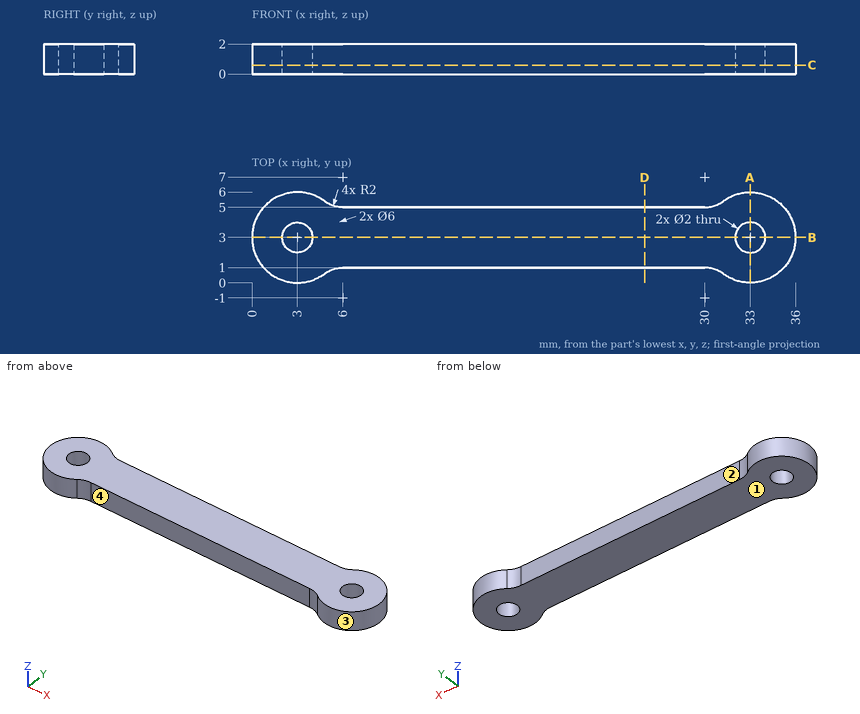
Job drawing, mm, ordinate dimensions from the low corner. One solid piece. A direction names the side the tool comes from. Coordinates: 2 decimals unless noted, no trailing zeros. Write each loop counter-clockwise with the first axis right and the second up, starting at its lowest first coordinate (ties: lowest second). Pieces come first, ordered by that corner, then holes. Notation, with made-up numbers: M -14.5,45 L 24.5,45 A21 cw 24.5,67 Z; hole C 72.25,-23 d9. An arc over 180 degrees is marked long. Answer as a JSON object with one key per item and string values. Group by question number.
1) Pin check, flat tips, straight feed: pin 1 Ø0.6 at (x, z) = (12.5, 1) entering from -Y; pin 2 Ø1 at (y, z) = (1, 0.5) entering from +X; pin 3 Ø1.8 at (x, y) = (33, 3) entering from +Z. Stop position of each tip, or through.
2) Saw through at A-A (x = 33). Write the cut outline in (y, z).
3) Mould opens along X. For the marked faces 1 and 2 say: +X half, -X half, draft (parallel to the pull), parting line (faces both ways), or undercut.
4) Wall check: line 1 (Y direction, x = 3, z = 1.3); line 2 (X direction, y = 3.5, z = 1.65); line 3 (X direction, y = 2.1, z = 1.3). Give the ranges that are in metal, low to high. Write a range as from..to.
5) Saw through at D-D (x = 26). Write the cut outline in (y, z).
6) Tool access for the marked faces 3 and 4: list every direction of +Z, -Z, +X, -X, +Y, -Y with a clear straight run to the whole face (end or side of a thin tool).
7) Saw through at B-B (y = 3). Write the cut outline in (x, z).
8) Saw through at C-C (z = 0.6). Write the cut outline in (x, y), plus the area to 3 significant figures.
Values follow:
{
 "1": {"pin 1": "stops at y = 1", "pin 2": "stops at x = 35.6", "pin 3": "passes through"},
 "2": {"outline": "M 0,0 L 2,0 L 2,2 L 0,2 Z; M 4,0 L 6,0 L 6,2 L 4,2 Z"},
 "3": {"face 1": "draft", "face 2": "undercut"},
 "4": {"line 1": "y = 0..2, 4..6", "line 2": "x = 0.04..2.13, 3.87..32.13, 33.87..35.96", "line 3": "x = 0.14..2.56, 3.44..32.56, 33.44..35.86"},
 "5": {"outline": "M 1,0 L 5,0 L 5,2 L 1,2 Z"},
 "6": {"face 3": "+Z, -Z", "face 4": "+Z, -Z, -Y"},
 "7": {"outline": "M 0,0 L 2,0 L 2,2 L 0,2 Z; M 4,0 L 32,0 L 32,2 L 4,2 Z; M 34,0 L 36,0 L 36,2 L 34,2 Z"},
 "8": {"outline": "M 4.8,0.6 A2 cw 6,1 L 30,1 A2 cw 31.2,0.6 A3 ccw long 31.2,5.4 A2 cw 30,5 L 6,5 A2 cw 4.8,5.4 A3 ccw long Z; hole C 3,3 d2; hole C 33,3 d2", "area": "148 mm2"}
}
